Can you work these out from the model? Positions are in its coordinate system, mm. A direction names the side the tool comes from. Give positions to 0.01 mm unless a question says otherwise; leave off trailing zeros. Loops run counter-clockwise (first coordinate to the right, second up) from the corner with the lowest first, then second, coordinate; pieces in that order, holes last. Notation, with made-up numbers: M 80,42.5 L 91,42.5 A31 ccw 91,68.5 Z; hole C -29,-19.75 d6. An arc over 180 degrees is marked long. Answer as a JSON object with one key per item and string values.
```python
from build123d import *

# Parameters (mm, degrees)
CHAMFER_1_SIZE = 0.5


with BuildPart() as part:
    # 草图1 → 旋转1 (revolve)
    with BuildSketch(Plane.XY, mode=Mode.PRIVATE) as revolve_1_sk:
        Polygon((-132.5, 4), (132.5, 4), (132.5, 3), (147.5, 3), (147.5, 2.75), (148, 2.75), (148, 3), (151, 3), (151, 0), (-158.5, 0), (-158.5, 3), (-148, 3), (-148, 2.75), (-147.5, 2.75), (-147.5, 3), (-132.5, 3), align=None)
    revolve(revolve_1_sk.sketch.rotate(Axis((0, 0, 0), (1, 0, 0)), 90), axis=Axis((0, 0, 0), (1, 0, 0)))

    # 倒角1
    chamfer_1_edges = [part.edges().sort_by_distance(p)[0] for p in [
        (151, 0, -3),
        (-158.5, 0, -3),
    ]]
    chamfer(chamfer_1_edges, length=CHAMFER_1_SIZE)


solid = part.part
```
1) Suppose I cut it at C-C, the plane x = -61. Write out the boundary of the cut face in (y, z).
Answer list:
{"outline": "C 0,0 d8"}
2) For faces 1 (the flat face through (132.5, -3, 1)), 2 (the cylindrical face through (-147.746, 2.685, -0.596)), 3 (the flat face through (-132.5, -3, -1)), 4 (the flat face through (151, 0, 0)), which set-ups out of +Z, -Z, +X, -X, +Y, -Y let a thin tool reach every point of the face, with its end or its side?
Answer list:
{"face 1": "+X", "face 2": "none", "face 3": "-X", "face 4": "+Z, -Z, +X, +Y, -Y"}
3) Will this pin go through, and if not, where does the flat tip stop? pin 1 Ø1.5 at (x, y) = (18.5, -1) entering from -Z.
Answer list:
{"pin 1": "z = -3.99"}
4) Please list where these lines run through material, in increasing order: line 1 along X through (y, z) = (-2.5, 2); line 2 along X through (y, z) = (2, -2); line 3 along Y through (x, z) = (102, 0.25). Write a range as from..to.
Answer list:
{"line 1": "-132.5..132.5", "line 2": "-158.17..-148, -147.5..147.5, 148..150.67", "line 3": "-3.99..3.99"}
5) If we mould it in two halves opening along X, with no side actions, what happens to faces 5 (the cylindrical face through (147.754, 2.685, -0.596)), 6 (the flat face through (-158.5, 0, 0)), 7 (the cylindrical face through (1.855, 3.905, -0.867))? For each: +X half, -X half, draft (parallel to the pull), parting line (faces both ways), or undercut.
Answer list:
{"face 5": "undercut", "face 6": "-X half", "face 7": "draft"}
